Input: part model. Units: mm. Frame: model coordinates. Face numbers are marked on the shaded views. A direction names the side the tool comes from. Round coordinates to 2 decimals unless told otherwise and drop trailing zeros. Loops run counter-clockwise (first coordinate to the right, second up) from the corner with the lowest first, then second, coordinate; pieces in that order, holes last. Notation, with made-up numbers: M -20,-25.75 L 10,-25.75 A18 ccw 10,0.25 Z; hole C 69.25,3 d1. An arc over 180 degrees is marked long. Put each result on its own line as item: value. Start each with the question number.
1) Pin query (flat end, axial travel): pin 1 (1.5 mm diameter, centred on y = -9, z = 11, fed in from +X); pin 2 (10 mm diameter, centred on y = 10, z = -63, fed in from -X); pin 3 (4 mm diameter, centred on x = 12.5, y = -5.5, fed in from +Z); pin 4 (3 mm diameter, centred on x = -13, z = -36, fed in from -Y). Return the tip coordinate at first contact, or that it passes through.
2) Section A-A on z = 5. Output: boundary loops of the cut face in (x, y), plus the area to 3 significant figures.
3) Reachability of the marked faces 4 and 5 from +Z, -Z, +X, -X, +Y, -Y: full face, straight path, thin tool, end or side. Return the list, or none.
4) Line query: probe 1 along Y at (x, z) = (0, 78); probe 2 along Z at (x, y) = (-10, -1); probe 3 along Z at (x, y) = (0.5, 3). Output: solid intervals per line, ascending.
5) Draft query along Z for the marked faces 1, 2 and 3. Return one class per face: +Z half, -Z half, draft (parallel to the pull), parting line (faces both ways), or undercut.
from build123d import *

# Parameters (mm, degrees)
SKETCH_1_R      = 10
EXTRUDE_1_DEPTH = 58.25
SKETCH_2_R      = 13.5
EXTRUDE_2_DEPTH = 16.5
EXTRUDE_START   = 14
SKETCH_3_R      = 10
EXTRUDE_3_DEPTH = 14
SKETCH_4_R      = 3
EXTRUDE_4_DEPTH = 0.48
SKETCH_5_R      = 9
EXTRUDE_5_DEPTH = 23.5
CHAMFER_1_SIZE  = 4
SKETCH_6_R      = 17.25
SKETCH_6_R_2    = 10.5
EXTRUDE_6_DEPTH = 3
EXTRUDE_7_DEPTH = 8
CHAMFER_2_SIZE  = 3
EXTRUDE_START_2 = 3
SKETCH_8_R      = 17.25
EXTRUDE_8_DEPTH = 3
EXTRUDE_9_DEPTH = 8


with BuildPart() as part:
    # Sketch 1 → Extrude 1 (new, symmetric)
    with BuildSketch(Plane.XY):
        Circle(SKETCH_1_R)
    extrude(amount=EXTRUDE_1_DEPTH, both=True)

    # Sketch 2 → Extrude 2 (add)
    with BuildSketch(Plane.XY.offset(58.25)):
        Circle(SKETCH_2_R)
    extrude_2 = extrude(amount=EXTRUDE_2_DEPTH)

    # Sketch 3 → Extrude 3 (add)
    with BuildSketch(Plane.XY.offset(74.75).offset(EXTRUDE_START)):
        Circle(SKETCH_3_R)
    extrude_3 = extrude(amount=-EXTRUDE_3_DEPTH)

    # Sketch 4 → Extrude 4 (add)
    with BuildSketch(Plane.XY.offset(88.75)):
        Circle(SKETCH_4_R)
    extrude_4 = extrude(amount=EXTRUDE_4_DEPTH)

    # Sketch 5 → Extrude 5 (add)
    with BuildSketch(Plane.XY.offset(89.23)):
        Circle(SKETCH_5_R)
    extrude_5 = extrude(amount=EXTRUDE_5_DEPTH)

    # Chamfer 1
    chamfer_1_edges = [part.edges().sort_by_distance(p)[0] for p in [
        (-9, 0, 112.73),
    ]]
    chamfer(chamfer_1_edges, length=CHAMFER_1_SIZE)



with BuildPart() as body_2:
    # Sketch 6 → Extrude 6 (new body)
    with BuildSketch(Plane.XY.offset(76.75)):
        Circle(SKETCH_6_R)
        Circle(SKETCH_6_R_2, mode=Mode.SUBTRACT)
    extrude(amount=EXTRUDE_6_DEPTH)


with BuildPart() as part_1:
    add(part.part)

    add(body_2.part)  # Extrude 7 merges body 2
    # Sketch 7 → Extrude 7 (add)
    with BuildSketch(Plane.XY.offset(79.75)):
        Polygon((6.392369232, 14.217510879), (-9.116540984, 12.644709585), (-15.508910216, -1.572801294), (-6.392369232, -14.217510879), (9.116540984, -12.644709585), (15.508910216, 1.572801294), align=None)
    extrude(amount=EXTRUDE_7_DEPTH)

    # Mirror 3: Extrude 2, Extrude 3, Extrude 4, Extrude 5 across plane
    add(extrude_2.mirror(Plane.XY))
    add(extrude_3.mirror(Plane.XY))
    add(extrude_4.mirror(Plane.XY))
    add(extrude_5.mirror(Plane.XY))

    # Chamfer 2
    chamfer_2_edges = [part_1.edges().sort_by_distance(p)[0] for p in [
        (-9, 0, -112.73),
    ]]
    chamfer(chamfer_2_edges, length=CHAMFER_2_SIZE)

    # Sketch 8 → Extrude 8 (add)
    with BuildSketch(Plane(origin=(0, 0, -76.75), x_dir=(-1, 0, 0), z_dir=(0, 0, -1)).offset(EXTRUDE_START_2)):
        with Locations(Location((0, 0, 0), (0, 0, 180))):
            Circle(SKETCH_8_R)
    extrude(amount=-EXTRUDE_8_DEPTH)

    # Sketch 9 → Extrude 9 (add)
    with BuildSketch(Plane(origin=(0, 0, -79.75), x_dir=(-1, 0, 0), z_dir=(0, 0, -1))):
        Polygon((7.878667531, 14.115945993), (-8.285434063, 13.881099226), (-16.164101594, -0.234846767), (-7.878667531, -14.115945993), (8.285434063, -13.881099226), (16.164101594, 0.234846767), align=None)
    extrude(amount=EXTRUDE_9_DEPTH)


solid = part_1.part
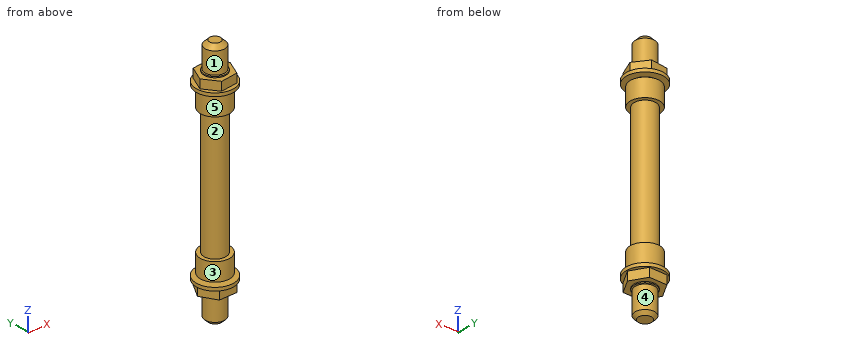
Geometry results:
1. pin 1: stops at x = 5.65
1. pin 2: stops at x = -12.54
1. pin 3: stops at z = 87.75
1. pin 4: passes through
2. outline: C 0,0 d20
2. area: 314 mm²
3. face 4: -Z
3. face 5: none
4. probe 1: y = -17.25 to -10.5, -10 to 10, 10.5 to 17.25
4. probe 2: z = -87.75 to -76.75, -74.75 to -58.25, 58.25 to 74.75, 79.75 to 87.75
4. probe 3: z = -112.73 to -89.23, -88.75 to 88.75, 89.23 to 112.73
5. face 1: draft
5. face 2: undercut
5. face 3: undercut
